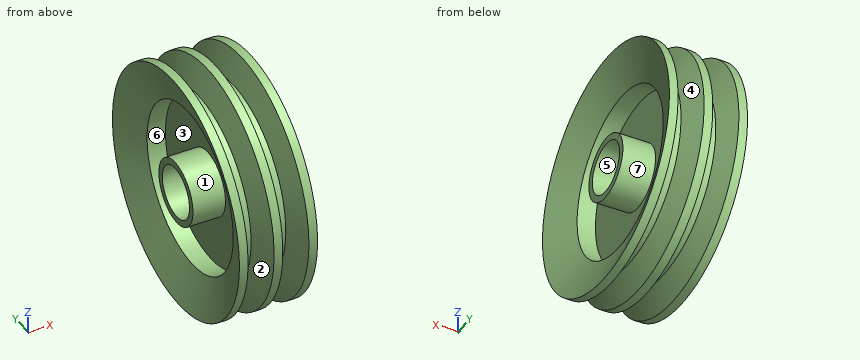
```python
from build123d import *


with BuildPart() as part:
    # Croquis1 → Revolución1 (revolve)
    with BuildSketch(Plane(origin=(0, 0, 0), x_dir=(1, 0, 0), z_dir=(0, 1, 0)), mode=Mode.PRIVATE) as revoluci_n1_sk:
        Polygon((-5, 110), (5, 110), (15.919107028, 80), (24.080892972, 80), (35, 110), (45, 110), (28.621339458, 65), (7.5, 65), (7.5, 7.5), (45, 7.5), (45, 0), (-45, 0), (-45, 7.5), (-7.5, 7.5), (-7.5, 65), (-28.621339458, 65), (-45, 110), (-35, 110), (-24.080892972, 80), (-15.919107028, 80), align=None)
    revolve(revoluci_n1_sk.sketch.rotate(Axis((-45, 0, 30), (1, 0, 0)), 180), axis=Axis((-45, 0, 30), (1, 0, 0)))


solid = part.part
```
Verification items for the finished model (mm, model axes). Face numbers are marked on the shaded views. A direction names the side the tool comes from. Coordinates: 2 decimals unless noted, no trailing zeros. Loops run counter-clockwise (first coordinate to the right, second up) from the corner with the lowest first, then second, coordinate; pieces in that order, holes last. Notation, with made-up numbers: (5.5, 84) - (13.5, 84) arc R22 ccw to (13.5, 103) - close; hole circle Ø10 at (66, -32). An arc over 180 degrees is marked (long way). Answer as a JSON object with one key per item and string values.
(1) Access from +Z, -Z, +X, -X, +Y, -Y to the whole of each face (thin tool, end or side, straight path). Record for the marked faces 4, 5, 6 and 7.
Response:
{"face 4": "none", "face 5": "+X, -X", "face 6": "-X", "face 7": "+X"}
(2) Cross-section at A-A, the plane x = 11.5. Record the boundary of the cut face in (y, z).
Response:
{"outline": "circle Ø244.28 at (0, 30); circle Ø75 at (0, 30); hole circle Ø190 at (0, 30); hole circle Ø60 at (0, 30)"}
(3) Scan lines: line 1 along Y through (x, z) = (-20.75, 30); line 2 along Y through (x, z) = (-1.5, 30); line 3 along X through (y, z) = (114.5, 7.5). Record each from-to range of solid material in increasing order.
Response:
{"line 1": "y = -110 to -95, -37.5 to -30, 30 to 37.5, 95 to 110", "line 2": "y = -140 to -30, 30 to 140", "line 3": "x = -36.52 to -26.52, -13.48 to 13.48, 26.52 to 36.52"}
(4) Go/stop test with flat-tipped pins: pin 1 Ø1 at (x, z) = (35.5, 49) entering from +Y; pin 2 Ø6 at (y, z) = (-23, 92) entering from +X; pin 3 Ø3 at (x, z) = (21.5, 101.5) entering from -Y. Record where each tip stops, or that it passes through.
Response:
{"pin 1": "stops at y = 138.77", "pin 2": "stops at x = 7.5", "pin 3": "stops at y = -84.85"}
(5) Mould release check, pull along X, two halves, no side actions. Record for the marked faces 1, 2 and 3: pulls with the +X half, pulls with the -X half, needs draft (parallel to the pull), parting line crosses it, or undercut.
Response:
{"face 1": "needs draft", "face 2": "undercut", "face 3": "pulls with the -X half"}
